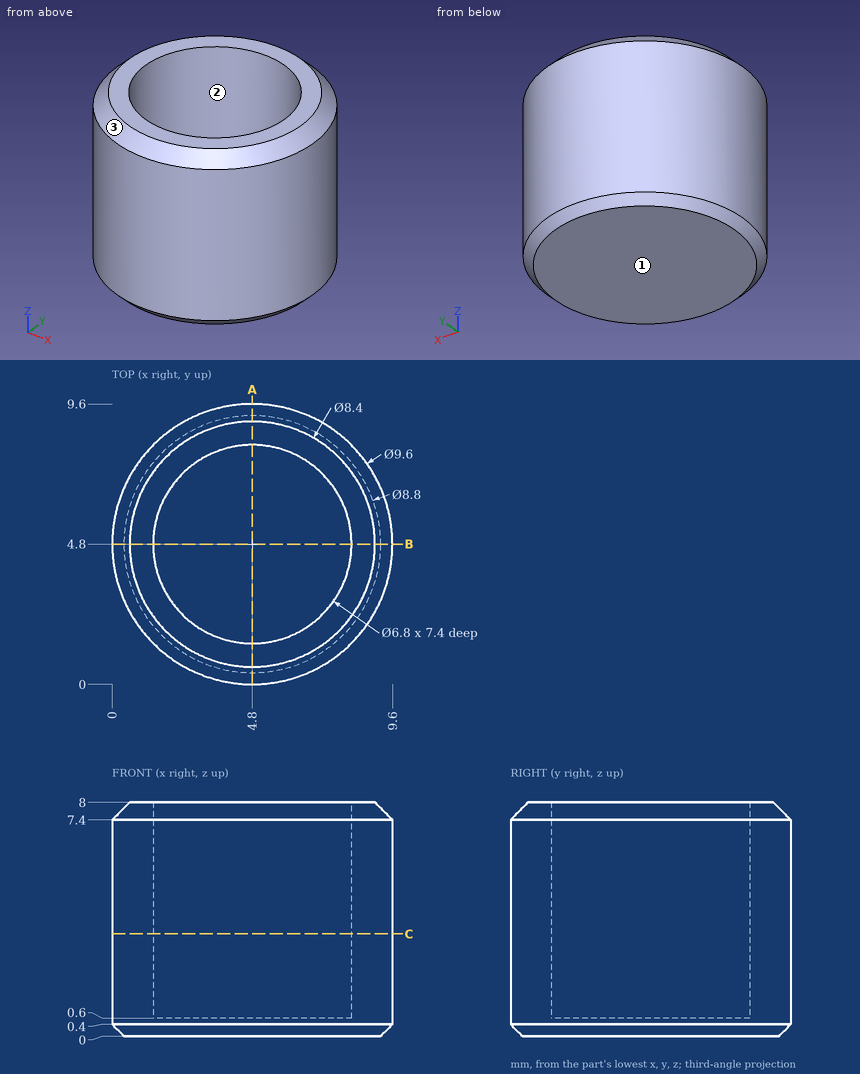
Print and shaded views of the part. All mm, measured from the part's lowest x, y and z. Give positions to 0.01 mm unless a question says otherwise; leave off trailing zeros. Order: outer loops, then holes, each group sorted by start corner. A loop starts at its lowest first (then second) coordinate and runs counter-clockwise, first axis right, second up. Notation, with made-up numbers: (-8, 61) -> (51, 61) arc R24 ccw to (51, 83) -> close; hole circle Ø8 at (-34.5, 16.25). An arc over 180 degrees is marked (long way). Use CSV: the item, a comma, the result in double quotes.
1. Band-saw the part on C-C, the plane z = 3.5. Give the cut face in (x, y).
Outcome:
outline,"circle Ø9.6 at (4.8, 4.8); hole circle Ø6.8 at (4.8, 4.8)"
2. Band-saw the part on A-A, the plane x = 4.8. Give the cut face in (y, z), then the cut area to 3 significant figures.
Outcome:
outline,"(0, 0.4) -> (0.4, 0) -> (9.2, 0) -> (9.6, 0.4) -> (9.6, 7.4) -> (9, 8) -> (8.2, 8) -> (8.2, 0.6) -> (1.4, 0.6) -> (1.4, 8) -> (0.6, 8) -> (0, 7.4) -> close"
area,"26.0 mm²"
3. Drill centre lines: line 1 along Y through (x, z) = (4.8, 2.25); line 2 along Z through (x, y) = (4.5, 7); line 3 along X through (y, z) = (4.5, 4.75). Where is each one in solid material? Low to high. Write a range as from..to.
Outcome:
line 1,"0..1.4, 8.2..9.6"
line 2,"0..0.6"
line 3,"0.01..1.41, 8.19..9.59"
4. Mould opens along X. For the marked faces 1, 2 and 3 say: +X half, -X half, draft (parallel to the pull), parting line (faces both ways), or undercut.
Outcome:
face 1,"draft"
face 2,"undercut"
face 3,"parting line"
5. Drop flat-ended pins along their axis: pin 1 (5 mm diameter, centred on x = 4, y = 5.5, fed in from +Z); pin 2 (4 mm diameter, centred on y = 7.5, z = 5.5, fed in from +X); pin 3 (1 mm diameter, centred on x = 2.5, z = 1, fed in from +Y); pin 4 (1 mm diameter, centred on x = 3, y = 6, fed in from +Z). Give the stop position or say it passes through.
Outcome:
pin 1,"z = 8"
pin 2,"x = 9.55"
pin 3,"y = 9.25"
pin 4,"z = 0.6"
